Can you work these out from the drawing? Everything is in mm from the part's minimum corner. A direction names the side the tool comes from. Round coordinates to 2 decimals unless told otherwise and drop trailing zeros. Loops run counter-clockwise (first coordinate to the right, second up) from the corner with the lowest first, then second, coordinate; pieces in that order, holes last. Notation, with made-up numbers: (-4, 27.25) -> (36, 27.25) arc R20 ccw to (36, 31.25) -> close; hole circle Ø1 at (20, -5.75). An arc over 180 degrees is marked (long way). One line per item, written item: value.
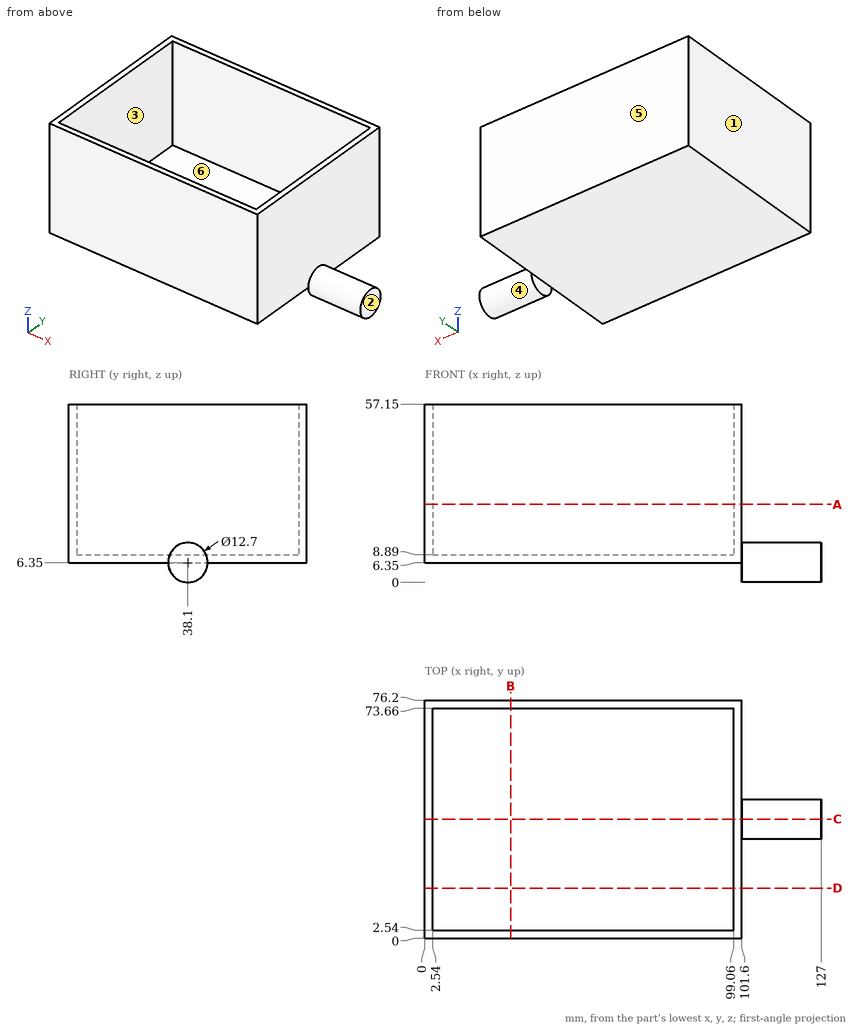
Item 1: If we section it at B-B on x = 27.5: List the corners of the cut face in (y, z) for me, plus the area to 3 significant figures.
Output:
outline: (0, 6.35) -> (76.2, 6.35) -> (76.2, 57.15) -> (73.66, 57.15) -> (73.66, 8.89) -> (2.54, 8.89) -> (2.54, 57.15) -> (0, 57.15) -> close
area: 439 mm²
Item 2: For the marked faces 4, 5 and 6, which set-ups out of +Z, -Z, +X, -X, +Y, -Y let a thin tool reach every point of the face, with its end or its side?
Output:
face 4: +X
face 5: +Z, -Z, +X, -X, +Y
face 6: +Z
Item 3: If we mould it in two halves opening along X, with no side actions, what happens to the marked faces 1, 2 and 3? For each: released by +X, released by -X, zero draft, split by the parting line, or undercut.
Output:
face 1: released by -X
face 2: released by +X
face 3: undercut
Item 4: Will these pins go through, and if not, where does the flat tip stop? pin 1 Ø12 at (x, y) = (91.5, 46) entering from -Z; pin 2 Ø1.5 at (y, z) = (63, 28) entering from +X; pin 3 Ø5 at (y, z) = (41, 3.5) entering from -X.
Output:
pin 1: stops at z = 6.35
pin 2: stops at x = 101.6
pin 3: stops at x = 101.6
Item 5: If we section it at D-D on y = 16: List the corners of the cut face in (x, z) for me, plus the area to 3 significant figures.
Output:
outline: (0, 6.35) -> (101.6, 6.35) -> (101.6, 57.15) -> (99.06, 57.15) -> (99.06, 8.89) -> (2.54, 8.89) -> (2.54, 57.15) -> (0, 57.15) -> close
area: 503 mm²
Item 6: If we section it at A-A on z = 25: List the corners of the cut face in (x, y) for me.
Output:
outline: (0, 0) -> (101.6, 0) -> (101.6, 76.2) -> (0, 76.2) -> close; hole (2.54, 2.54) -> (99.06, 2.54) -> (99.06, 73.66) -> (2.54, 73.66) -> close
Item 7: If we section it at C-C on y = 38.1: List the corners of the cut face in (x, z) for me.
Output:
outline: (0, 6.35) -> (101.6, 6.35) -> (101.6, 0) -> (127, 0) -> (127, 12.7) -> (101.6, 12.7) -> (101.6, 57.15) -> (99.06, 57.15) -> (99.06, 8.89) -> (2.54, 8.89) -> (2.54, 57.15) -> (0, 57.15) -> close
Item 8: I need wall thicknesses on line 1 (X direction, y = 19.5, z = 55.5); line 2 (Y direction, x = 13.5, z = 45); line 3 (Z direction, x = 35, y = 68). Which ranges of each line are inside material? Lowest first, please. Write a range as from..to.
Output:
line 1: x = 0..2.54, 99.06..101.6
line 2: y = 0..2.54, 73.66..76.2
line 3: z = 6.35..8.89
